Design review of the part built by this model. Coordinates are the model's own, in mm. A direction names the side the tool comes from. Coordinates: 2 decimals unless noted, no trailing zeros. Loops run counter-clockwise (first coordinate to the right, second up) from the corner with the lowest first, then second, coordinate; pieces in that order, holes last. Notation, with made-up numbers: M -31.75,57 L -20.75,57 A19 cw -20.75,76 Z; hole C 33,-32.75 d7. An arc over 180 degrees is marked long. Write item = value, one per line. Start each with the question number.
```python
from build123d import *

# Parameters (mm, degrees)
F0_W     = 19
F0_H     = 9
F1_DEPTH = 5
F3_D     = 4.2
F5_D     = 6
F7_D     = 2.5
F7_DEPTH = 5
F7_TIP   = 0.7510757738
F9_D     = 2.5
F9_DEPTH = 6
F9_TIP   = 0.7510757738


with BuildPart() as f1:
    # F0 (on Top) → F1 (new body, symmetric)
    with BuildSketch(Plane.XY):
        Rectangle(F0_W, F0_H)
    extrude(amount=F1_DEPTH, both=True)

    # F3 (through all)
    with Locations(Plane.XY.offset(5)):
        with Locations((-3.5, 0)):
            Hole(F3_D / 2)

    # F5 (through all)
    with Locations(Plane.XZ.offset(4.5)):
        with Locations((3.5, 0)):
            Hole(F5_D / 2)

    # F7
    with Locations(Plane.YZ.offset(9.5)):
        with Locations((0, 0)):
            Hole(F7_D / 2, depth=F7_DEPTH)
            with Locations((0, 0, -(F7_DEPTH + F7_TIP / 2))):  # 118° drill point
                Cone(0, F7_D / 2, F7_TIP, mode=Mode.SUBTRACT)

    # F9
    with Locations(Plane(origin=(-9.5, 0, 0), x_dir=(0, -1, 0), z_dir=(-1, 0, 0))):
        with Locations((0, 0)):
            Hole(F9_D / 2, depth=F9_DEPTH)
            with Locations((0, 0, -(F9_DEPTH + F9_TIP / 2))):  # 118° drill point
                Cone(0, F9_D / 2, F9_TIP, mode=Mode.SUBTRACT)


solid = f1.part
```
(1) Tool access review of faces 1 (the cylindrical face through (7.84, 0.16, 1.24)), 2 (the cylindrical face through (-7.31, -1.25, 0.05)), 3 (the cylindrical face through (-1.4, 0.09, -0.07)): name each direction out of +Z, -Z, +X, -X, +Y, -Y from which nothing blocks a thin tool from reaching the whole face with its end or side.
(2) Take a section at B-B (z = 0). State the section outline as (x, y) points.
(3) Take a section at C-C (x = 3.5). State the section outline as (y, z) points, plus the area to 3 significant figures.
(4) Mouldability with a two-part tool opening along X and no side actions: class faces 4 (the cylindrical face through (0.73, 0.06, -1.15)), 5 (the flat face through (9.5, -1, -1)), 6 (the flat face through (0, 0, -5)) as +X half, -X half, draft (parallel to the pull), parting line (faces both ways), or undercut.
(5) Take a section at A-A (y = 0). State the section outline as (x, z) points, plus the area to 3 significant figures.
(6) To check wall thickness, follow L1, parallel to Y at x = -3.5, z = 1.25; L2, parallel to Z at x = -8.3, y = 0; L3, parallel to Y at x = 7.6, z = 0. State the ranges of each line that lie inside material, in increasing order.
(7) Take a section at D-D (x = -6.75). State the section outline as (y, z) points, plus the area to 3 significant figures.
Results list:
q1.face_1 = +X
q1.face_2 = -X
q1.face_3 = +Z, -Z
q2.outline = M -9.5,-4.5 L 0.5,-4.5 L 0.5,4.5 L -9.5,4.5 L -9.5,1.25 L -5.19,1.25 A2.1 cw long -5.19,-1.25 L -9.5,-1.25 Z; M 6.5,-4.5 L 9.5,-4.5 L 9.5,-1.25 L 6.5,-1.25 Z; M 6.5,1.25 L 9.5,1.25 L 9.5,4.5 L 6.5,4.5 Z
q3.outline = M -4.5,-5 L 4.5,-5 L 4.5,-3 L -4.5,-3 Z; M -4.5,3 L 4.5,3 L 4.5,5 L -4.5,5 Z
q3.area = 36.0 mm^2
q4.face_4 = undercut
q4.face_5 = +X half
q4.face_6 = draft
q5.outline = M -9.5,-5 L -5.6,-5 L -5.6,-1.25 L -9.5,-1.25 Z; M -9.5,1.25 L -5.6,1.25 L -5.6,5 L -9.5,5 Z; M -1.4,-5 L 9.5,-5 L 9.5,-1.25 L 6.23,-1.25 A3 cw long 6.23,1.25 L 9.5,1.25 L 9.5,5 L -1.4,5 Z
q5.area = 102 mm^2
q6.L1 = -4.5 to -2.1, 2.1 to 4.5
q6.L2 = -5 to -1.25, 1.25 to 5
q6.L3 = -4.5 to -1.25, 1.25 to 4.5
q7.outline = M -4.5,-5 L 4.5,-5 L 4.5,5 L -4.5,5 Z; hole C 0,0 d2.5
q7.area = 85.1 mm^2
